from build123d import *

# Parameters (mm, degrees)
F0_R     = 1.18
F1_DEPTH = 0.2


with BuildPart() as f1:
    # F0 (on Top) → F1 (new body)
    with BuildSketch(Plane.XY):
        with BuildLine():
            Line((2.338535, -12.207578), (3.923982, -0.532885))
            ThreePointArc((3.923982, -0.532885), (0, 3.96), (-3.923982, -0.532885))
            Line((-3.923982, -0.532885), (-2.338535, -12.207578))
            ThreePointArc((-2.338535, -12.207578), (0, -14.25), (2.338535, -12.207578))
        make_face()
        with Locations((0, -11.89)):
            Circle(F0_R, mode=Mode.SUBTRACT)
        with Locations((0, -8.71)):
            Circle(F0_R, mode=Mode.SUBTRACT)
        with BuildLine():
            ThreePointArc((-1.078338, -1.078338), (-1.320689, -0.7625), (-1.473037, -0.394699))
            Line((-1.473037, -0.394699), (-2.656296, -0.711752))
            ThreePointArc((-2.656296, -0.711752), (-2.75, 0), (-2.656296, 0.711752))
            Line((-2.656296, 0.711752), (-1.473037, 0.394699))
            ThreePointArc((-1.473037, 0.394699), (-1.320689, 0.7625), (-1.078338, 1.078338))
            Line((-1.078338, 1.078338), (-1.944544, 1.944544))
            ThreePointArc((-1.944544, 1.944544), (-1.375, 2.38157), (-0.711752, 2.656296))
            Line((-0.711752, 2.656296), (-0.394699, 1.473037))
            ThreePointArc((-0.394699, 1.473037), (0, 1.525), (0.394699, 1.473037))
            Line((0.394699, 1.473037), (0.711752, 2.656296))
            ThreePointArc((0.711752, 2.656296), (1.375, 2.38157), (1.944544, 1.944544))
            Line((1.944544, 1.944544), (1.078338, 1.078338))
            ThreePointArc((1.078338, 1.078338), (1.320689, 0.7625), (1.473037, 0.394699))
            Line((1.473037, 0.394699), (2.656296, 0.711752))
            ThreePointArc((2.656296, 0.711752), (2.75, 0), (2.656296, -0.711752))
            Line((2.656296, -0.711752), (1.473037, -0.394699))
            ThreePointArc((1.473037, -0.394699), (1.320689, -0.7625), (1.078338, -1.078338))
            Line((1.078338, -1.078338), (1.944544, -1.944544))
            ThreePointArc((1.944544, -1.944544), (1.375, -2.38157), (0.711752, -2.656296))
            Line((0.711752, -2.656296), (0.394699, -1.473037))
            ThreePointArc((0.394699, -1.473037), (0, -1.525), (-0.394699, -1.473037))
            Line((-0.394699, -1.473037), (-0.711752, -2.656296))
            ThreePointArc((-0.711752, -2.656296), (-1.375, -2.38157), (-1.944544, -1.944544))
            Line((-1.944544, -1.944544), (-1.078338, -1.078338))
        make_face(mode=Mode.SUBTRACT)
    extrude(amount=F1_DEPTH)


solid = f1.part
Part model, mm, in its own coordinate system. Coordinates: 2 decimals unless noted, no trailing zeros. Order: outer loops, then holes, each group sorted by start corner. A loop starts at its lowest first (then second) coordinate and runs counter-clockwise, first axis right, second up.
(1) Slice it at C-C, the plane x = -1.75. Write the cut outline in (y, z).
Check sheet entries:
outline: (-13.47, 0) - (-2.12, 0) - (-2.12, 0.2) - (-13.47, 0.2) - close; (-1.75, 0) - (-0.47, 0) - (-0.47, 0.2) - (-1.75, 0.2) - close; (0.47, 0) - (1.75, 0) - (1.75, 0.2) - (0.47, 0.2) - close; (2.12, 0) - (3.55, 0) - (3.55, 0.2) - (2.12, 0.2) - close
(2) Slice it at D-D, the plane x = 0. Write the cut outline in (y, z) (3 decimals).
Check sheet entries:
outline: (-14.25, 0) - (-13.07, 0) - (-13.07, 0.2) - (-14.25, 0.2) - close; (-10.71, 0) - (-9.89, 0) - (-9.89, 0.2) - (-10.71, 0.2) - close; (-7.53, 0) - (-1.525, 0) - (-1.525, 0.2) - (-7.53, 0.2) - close; (1.525, 0) - (3.96, 0) - (3.96, 0.2) - (1.525, 0.2) - close
(3) Probe L1, parallel to Y at x = 1.75, z = 0.15; L2, parallel to X at y = -11, z = 0.05; L3, parallel to X at y = -3.75, z = 0.1. List the from-to ranges inside material, lowest first.
Check sheet entries:
L1: y = -13.47 to -2.12, -1.75 to -0.47, 0.47 to 1.75, 2.12 to 3.55
L2: x = -2.5 to -0.77, 0.77 to 2.5
L3: x = -3.49 to 3.49
(4) Slice it at A-A, the plane y = 0. Write the cut outline in (x, z).
Check sheet entries:
outline: (-3.96, 0) - (-2.75, 0) - (-2.75, 0.2) - (-3.96, 0.2) - close; (2.75, 0) - (3.96, 0) - (3.96, 0.2) - (2.75, 0.2) - close
(5) Slice it at B-B, the plane z = 0.1. State how many separate pieces and enclosed holes the cut face has, and give its area (3 significant figures).
Check sheet entries:
separate pieces: 1
enclosed holes: 3
area: 84.9 mm2
